Read the model definition and answer for the solid it produces. Units are mm, in the model's axes. Face numbers are marked on the shaded views. Coordinates: 2 decimals unless noted, no trailing zeros. Loops run counter-clockwise (first coordinate to the right, second up) from the corner with the lowest first, then second, coordinate; pieces in that order, holes last. Notation, with made-up numbers: (87.5, 86) -> (92.5, 86) arc R9 ccw to (92.5, 92) -> close; hole circle Ø9 at (59.5, -31). An arc over 180 degrees is marked (long way). Answer as a JSON object with one key per item and string values. Group by question number.
Q1. The part is cut by section C-C on x = 68.5. Write down the section's boundary in (y, z), and give its area (3 significant figures).
Q2. Each of these flat-tipped pins is pushed along its axis until it touches: P1, Ø0.5, axis at x = 81.5, z = 2, coming from the +Y side; P2, Ø1.2, axis at x = 90.35, y = -50.5, coming from the +Z side; P3, Ø0.8, axis at y = -13, z = 2, coming from the +X side. Where does it stop, or does it pass through?
Q3. Determine the mould class of the marked faces 1 and 2 for opening direction X: released by +X, released by -X, zero draft, split by the parting line, or undercut.
Q4. Straight lines are drawn through the part: line 1 along Y through (x, z) = (24.5, 2.25); line 2 along Y through (x, z) = (50, 0.5); line 3 along Z through (x, y) = (82.5, -27). For each, find the intervals that lie inside material, in ascending order. Write a range as [from, to].
Q5. The part is cut by section A-A on x = 47. Write down the section's boundary in (y, z), and give its area (3 significant figures).
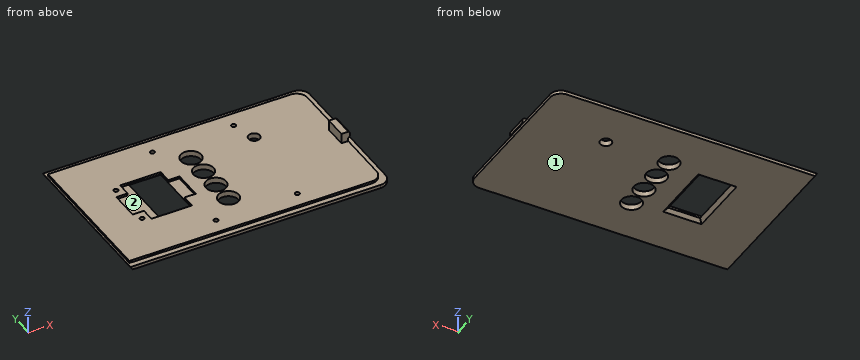
Autodesk Inventor part; units mm, degrees
ref_plane "YZ Plane" through (0, 0, 0) normal (1, 0, 0) x (0, 1, 0)
ref_plane "XZ Plane" through (0, 0, 0) normal (0, 1, 0) x (-1, 0, 0)
ref_plane "XY Plane" through (0, 0, 0) normal (0, 0, 1) x (1, 0, 0)
sketch "Skizze1" plane through (0, 0, 0) normal (0, 0, 1) x (1, 0, 0)
  line L0 (11.1165, 10) -> (126.7755, 10)
  line L1 (126.7755, 10) -> (126.7755, -60)
  line L2 (126.7755, -60) -> (11.1165, -60)
  line L3 (11.1165, -60) -> (11.1165, 10)
  line L4 (36.6476, -12.5) -> (50.6476, -12.5)
  line L5 (50.6476, -12.5) -> (50.6476, -37.5)
  line L6 (50.6476, -37.5) -> (36.6476, -37.5)
  line L7 (36.6476, -37.5) -> (36.6476, -12.5)
  line L8 (126.7755, -25) -> (11.1165, -25)
  line L9 (126.7755, -36.2282) -> (128.5882, -36.2282)
  line L10 (128.5882, -36.2282) -> (128.5882, -13.7718)
  line L11 (128.5882, -13.7718) -> (126.7755, -13.7718)
  line L12 (126.7755, -13.7718) -> (126.7755, -36.2282)
  circle A0 centre (65.6476, -10) radius 4.5
  circle A1 centre (65.6476, -20) radius 4.5
  circle A2 centre (65.6476, -30) radius 4.5
  circle A3 centre (65.6476, -40) radius 4.5
  circle A4 centre (93.6476, -10) radius 2.5
  point P0 (0, 0)
  dimension "d0" = 115.659
  dimension "d1" = 70
  dimension "d2" = 25
  dimension "d3" = 14
  dimension "d65" = 9
  dimension "d66" = 9
  dimension "d67" = 9
  dimension "d68" = 9
  dimension "d69" = 10
  dimension "d70" = 10
  dimension "d71" = 10
  dimension "d73" = 10
  dimension "d74" = 15
  dimension "d75" = 25.5312
  dimension "d76" = 22.5
  dimension "d77" = 5
  dimension "d79" = 28
extrude "Extrusion1" add sketch "Skizze1" along normal blind 1.5 contours L0 L1 L8 L5 L4 L7 L3 | L8 L7 L6 L5 L1 L2 L3
sketch "Skizze2" plane through (0, 0, 1.5) normal (0, 0, 1) x (1, 0, 0)
  point P0 (0, 0)
sketch "Skizze3" plane through (0, 0, 1.5) normal (0, 0, 1) x (1, 0, 0)
  line L0 (126.7755, -60) -> (126.7755, 10)
  line L1 (124.2755, -30) -> (121.2755, -30)
  line L2 (121.2755, -30) -> (121.2755, -20)
  line L3 (121.2755, -20) -> (124.2755, -20)
  line L4 (124.2755, -20) -> (124.2755, -30)
  line L5 (126.7755, -25) -> (117.2329, -25)
  line L6 (135, -36) -> (135, -24)
  line L7 (11.1165, -60) -> (126.7755, -60)
  line L8 (126.7755, 10) -> (11.1165, 10)
  point P0 (0, 0)
  dimension "d6" = 10
  dimension "d62" = 2.5
  dimension "d63" = 3
extrude "Extrusion2" add sketch "Skizze3" along normal blind 5.5
sketch "Skizze4" plane through (124.2755, -54, 0) normal (1, 0, 0) x (0, 0, -1)
  line L0 (-7, 24) -> (-7, 36)
  line L1 (-1.5, 34) -> (-7, 34)
  line L2 (-7, 24) -> (-4, 24)
  line L3 (-4, 24) -> (-4, 34)
  line L4 (-4, 34) -> (-7, 34)
  line L5 (-7, 34) -> (-7, 24)
  line L6 (-1.5, -6) -> (-1.5, 64)
  point P0 (0, 54)
  point P1 (-1.5, 24)
  point P2 (-7, 34)
  dimension "d9" = 2.5
extrude "Extrusion3" add sketch "Skizze4" along normal blind 0.8
chamfer "Fase1" distance 0.75 angle 45 2 edges at (125.0755, -25, 7) (125.0755, -25, 4)
chamfer "Fase2" distance 1.5 angle 45 4 edges at (36.6476, -25, 0) (43.6476, -12.5, 0) (50.6476, -25, 0) (43.6476, -37.5, 0)
chamfer "Fase3" distance 1.5 angle 30 1 edges at (11.1165, -25, 0) measured on face at (11.1165, -13.3333, 0.5)
sketch "Skizze5" plane through (0, 0, 1.5) normal (0, 0, 1) x (1, 0, 0)
  line L0 (11.9825, 10) -> (11.9825, -60)
  line L1 (11.9825, 7.5) -> (124.2755, 7.5)
  line L2 (124.2755, 7.5) -> (124.2755, -57.5)
  line L3 (124.2755, -57.5) -> (11.9825, -57.5)
  line L4 (11.9825, -57.5) -> (11.9825, 7.5)
  line L5 (126.7755, -60) -> (126.7755, 10)
  line L6 (126.7755, 10) -> (11.1165, 10)
  line L7 (11.1165, 10) -> (11.1165, -60)
  line L8 (11.1165, -60) -> (126.7755, -60)
  line L9 (27.8476, -18.5) -> (55.8476, -18.5)
  line L10 (55.8476, -18.5) -> (55.8476, -31.5)
  line L11 (55.8476, -31.5) -> (27.8476, -31.5)
  line L12 (27.8476, -31.5) -> (27.8476, -18.5)
  line L13 (36.6476, -37.5) -> (36.6476, -12.5)
  line L14 (36.6476, -12.5) -> (50.6476, -12.5)
  line L15 (58.8722, -25) -> (36.6476, -25)
  line L16 (36.6476, -37.5) -> (50.6476, -37.5)
  line L17 (32.8476, -37.5) -> (50.8476, -37.5)
  line L18 (50.8476, -37.5) -> (50.8476, -12.5)
  line L19 (50.8476, -12.5) -> (32.8476, -12.5)
  line L20 (32.8476, -12.5) -> (32.8476, -37.5)
  line L21 (50.6476, -37.5) -> (36.6476, -37.5)
  line L22 (50.6476, -12.5) -> (50.6476, -37.5)
  circle A0 centre (93.6476, -10) radius 2.5
  circle A1 centre (65.6476, -10) radius 4.5
  circle A2 centre (65.6476, -20) radius 4.5
  circle A3 centre (65.6476, -30) radius 4.5
  circle A4 centre (65.6476, -40) radius 4.5
  point P0 (0, 0)
  point P1 (135, -24)
  point P2 (36.6476, -18.5)
  point P3 (36.6476, -31.5)
  point P4 (50.8476, -31.5)
  point P5 (50.6476, -37.5)
  point P6 (36.6476, -37.5)
  point P7 (32.8476, -31.5)
  point P8 (32.8476, -18.5)
  point P9 (36.6476, -12.5)
  point P10 (50.6476, -12.5)
  point P11 (50.8476, -18.5)
  point P12 (126.7755, -13.7718)
  dimension "d21" = 2.5
  dimension "d22" = 2.5
  dimension "d24" = 2.5
  dimension "d25" = 0.866
  dimension "d26" = 28
  dimension "d27" = 13
  dimension "d28" = 8.8
  dimension "d60" = 5
  dimension "d61" = 5
  dimension "d64" = 5.2
extrude "Extrusion5" add sketch "Skizze5" along normal blind 1 contours L1 L2 L3 L0
sketch "Skizze6" plane through (0, 0, 2.5) normal (0, 0, 1) x (1, 0, 0)
  line L0 (27.8476, -31.5) -> (27.8476, -18.5)
  line L1 (55.8476, -18.5) -> (55.8476, -31.5)
  line L2 (36.6476, -12.5) -> (50.6476, -12.5)
  line L3 (50.6476, -37.5) -> (36.6476, -37.5)
  point P0 (0, 0)
  point P1 (29.8476, -35.5)
  point P2 (29.8476, -14.5)
  point P3 (54.3476, -50.5)
  point P4 (54.3476, 0.5)
  point P5 (90.3476, -50.5)
  point P6 (90.3476, 0.5)
  dimension "d36" = 2
  dimension "d37" = 2
  dimension "d38" = 1.5
  dimension "d39" = 1.5
  dimension "d42" = 2
  dimension "d80" = 13
  dimension "d81" = 13
  dimension "d82" = 2
  dimension "d83" = 36
  dimension "d84" = 36
hole "Bohrung1" at (29.8476, -35.5, 2.5) at (29.8476, -14.5, 2.5) at (54.3476, -50.5, 2.5) at (54.3476, 0.5, 2.5) at (90.3476, -50.5, 2.5) at (90.3476, 0.5, 2.5) direction (0, 0, -1) diameter 2 depth 2.25
fillet "Rundung1" radius 4.75 4 edges at (126.7755, 10, 0.75) (126.7755, -60, 0.75) (124.2755, -57.5, 2) (124.2755, 7.5, 2)
properties part number "Case top"
Final values:
{
 "1": {"outline": "(-60, 0) -> (-43.48, 0) -> (-43.48, 2.5) -> (-57.5, 2.5) -> (-57.5, 1.5) -> (-60, 1.5) -> close; (-36.52, 0) -> (-33.48, 0) -> (-33.48, 2.5) -> (-36.52, 2.5) -> close; (-26.52, 0) -> (-23.48, 0) -> (-23.48, 2.5) -> (-26.52, 2.5) -> close; (-16.52, 0) -> (-13.48, 0) -> (-13.48, 2.5) -> (-16.52, 2.5) -> close; (-6.52, 0) -> (10, 0) -> (10, 1.5) -> (7.5, 1.5) -> (7.5, 2.5) -> (-6.52, 2.5) -> close", "area": "100 mm2"},
 "2": {"P1": "stops at y = 7.5", "P2": "stops at z = 0.25", "P3": "stops at x = 124.28"},
 "3": {"face 1": "zero draft", "face 2": "undercut"},
 "4": {"line 1": "y = [-57.5, 7.5]", "line 2": "y = [-60, -38.5], [-11.5, 10]", "line 3": "z = [0, 2.5]"},
 "5": {"outline": "(-60, 0) -> (-39, 0) -> (-37.5, 1.5) -> (-37.5, 2.5) -> (-57.5, 2.5) -> (-57.5, 1.5) -> (-60, 1.5) -> close; (-12.5, 1.5) -> (-11, 0) -> (10, 0) -> (10, 1.5) -> (7.5, 1.5) -> (7.5, 2.5) -> (-12.5, 2.5) -> close", "area": "105 mm2"}
}
